The listing builds one solid part. Answer for the finished solid, in the listing's coordinates (mm). Round coordinates to 2 decimals unless told otherwise and drop trailing zeros. Order: outer loops, then holes, each group sorted by start corner. A loop starts at its lowest first (then second) coordinate and runs counter-clockwise, first axis right, second up. Notation, with made-up numbers: M 83,64.5 L 136,64.5 A17 ccw 136,83.5 Z; hole C -19,-39 d6. An arc over 180 degrees is marked long. Put each result on its own line as item: value. Start each with the question number.
1. The part is cut by section C-C (x = 18.5). Give the vertices of the cut face in (y, z), then the cut area to 3 significant figures.
2. The part is cut by section D-D (x = 14). Give the vertices of the cut face in (y, z), then the cut area to 3 significant figures.
3. The part is cut by section B-B (y = 0.25). Give the vertices of the cut face in (x, z), then the cut area to 3 significant figures.
4. Consider line 1 (X direction, y = 0.35, z = 21); line 2 (Z direction, x = 21.5, y = 1.25); line 3 (Z direction, x = 17, y = 1.4). Determine where each line is inside the solid, lowest interval first.
5. The part is cut by section A-A (z = -5). Give the vertices of the cut face in (x, y).
from build123d import *

# Parameters (mm, degrees)
SKETCH1_W          = 20
SKETCH1_H          = 34
BASE_FLANGE1_DEPTH = 1.5
SKETCH2_W          = 31
SKETCH2_H          = 8
TAB1_DEPTH         = 1.5
SKETCH4_R          = 1.5
CUT_EXTRUDE1_DEPTH = 10
SKETCH5_R          = 1.5
CUT_EXTRUDE2_DEPTH = 10


# Sheet-metal steps are written as plain solids
with BuildPart() as part:
    # Sketch1 → Base-Flange1 (new body)
    with BuildSketch(Plane(origin=(0, 0, 0), x_dir=(1, 0, 0), z_dir=(0, 1, 0))):
        Rectangle(SKETCH1_W, SKETCH1_H)
    extrude(amount=BASE_FLANGE1_DEPTH)

    # Sketch2 → Tab1 (add)
    with BuildSketch(Plane(origin=(0, 1.5, 0), x_dir=(1, 0, 0), z_dir=(0, 1, 0))):
        with Locations((9.5, -21)):
            Rectangle(SKETCH2_W, SKETCH2_H)
        with Locations((9.5, 21)):
            Rectangle(SKETCH2_W, SKETCH2_H)
    extrude(amount=-TAB1_DEPTH)

    # Sketch4 → Cut-Extrude1 (cut)
    with BuildSketch(Plane(origin=(0, 1.5, 0), x_dir=(1, 0, 0), z_dir=(0, 1, 0))):
        with Locations(Location((-3, 5, 0), (0, 0, 270))):
            Circle(SKETCH4_R)
        with Locations(Location((3, 5, 0), (0, 0, 270))):
            Circle(SKETCH4_R)
    extrude(amount=-CUT_EXTRUDE1_DEPTH, mode=Mode.SUBTRACT)

    # Sketch5 → Cut-Extrude2 (cut)
    with BuildSketch(Plane(origin=(0, 1.5, 0), x_dir=(1, 0, 0), z_dir=(0, 1, 0))):
        with Locations(Location((21, 21, 0), (0, 0, 270))):
            Circle(SKETCH5_R)
        with Locations(Location((15, 21, 0), (0, 0, 270))):
            Circle(SKETCH5_R)
        with Locations(Location((15, -21, 0), (0, 0, 270))):
            Circle(SKETCH5_R)
        with Locations(Location((21, -21, 0), (0, 0, 270))):
            Circle(SKETCH5_R)
    extrude(amount=-CUT_EXTRUDE2_DEPTH, mode=Mode.SUBTRACT)


solid = part.part
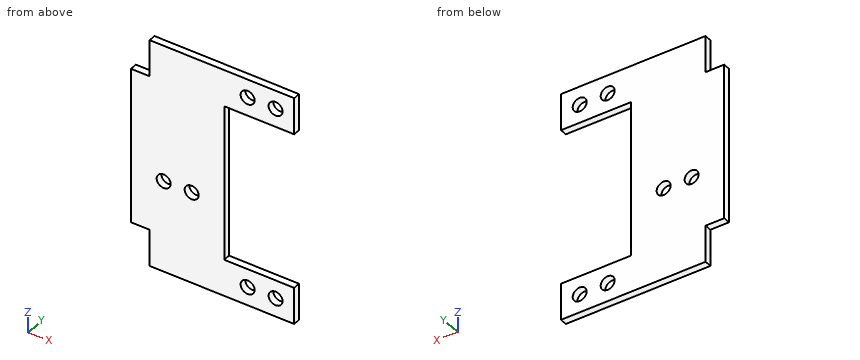
Resolved:
1. outline: M 0,-25 L 1.5,-25 L 1.5,-17 L 0,-17 Z; M 0,17 L 1.5,17 L 1.5,25 L 0,25 Z
1. area: 24.0 mm2
2. outline: M 0,-25 L 1.5,-25 L 1.5,-22.12 L 0,-22.12 Z; M 0,-19.88 L 1.5,-19.88 L 1.5,-17 L 0,-17 Z; M 0,17 L 1.5,17 L 1.5,19.88 L 0,19.88 Z; M 0,22.12 L 1.5,22.12 L 1.5,25 L 0,25 Z
2. area: 17.3 mm2
3. outline: M -10,-17 L -6,-17 L -6,-25 L 25,-25 L 25,-17 L 10,-17 L 10,17 L 25,17 L 25,25 L -6,25 L -6,17 L -10,17 Z; hole C -3,-5 d3; hole C 3,-5 d3; hole C 15,-21 d3; hole C 15,21 d3; hole C 21,-21 d3; hole C 21,21 d3
3. area: 1,130 mm2
4. line 1: -6 to 13.5, 16.5 to 19.5, 22.5 to 25
4. line 2: -25 to -22.41, -19.59 to -17, 17 to 19.59, 22.41 to 25
4. line 3: -25 to -17, 17 to 25
5. outline: M -10,0 L -4.5,0 L -4.5,1.5 L -10,1.5 Z; M -1.5,0 L 1.5,0 L 1.5,1.5 L -1.5,1.5 Z; M 4.5,0 L 10,0 L 10,1.5 L 4.5,1.5 Z
